For this review, take the finished solid that the model builds, in its own axes (mm). A direction names the side the tool comes from. Round coordinates to 2 decimals unless told otherwise and drop trailing zeros. Order: outer loops, then holes, each group sorted by start corner. A loop starts at its lowest first (then second) coordinate and runs counter-clockwise, first axis right, second up.
from build123d import *

# Parameters (mm, degrees)
BOSS_EXTRUDE1_DEPTH            = 8
CBORE_FOR_M5_SHCS1_D           = 5.5
CBORE_FOR_M5_SHCS1_DEPTH       = 8
CBORE_FOR_M5_SHCS1_CBORE_D     = 10.5
CBORE_FOR_M5_SHCS1_CBORE_DEPTH = 6


with BuildPart() as part:
    # Sketch1 → Boss-Extrude1 (new body)
    with BuildSketch(Plane(origin=(0, 0, 0), x_dir=(1, 0, 0), z_dir=(0, 1, 0))):
        with BuildLine():
            Line((3, 0), (37, 0))
            Line((37, 0), (40, 0))
            Line((40, 0), (40, 3))
            Line((40, 3), (40, 16))
            Line((40, 16), (25, 16))
            Line((25, 16), (25, 19))
            ThreePointArc((25, 19), (24.707106781, 19.707106781), (24, 20))
            Line((24, 20), (0, 20))
            Line((0, 20), (0, 3))
            ThreePointArc((0, 3), (0.878679656, 0.878679656), (3, 0))
        make_face()
    extrude(amount=BOSS_EXTRUDE1_DEPTH)

    # CBORE for M5 SHCS1
    with Locations(Plane(origin=(0, 8, 0), x_dir=(1, 0, 0), z_dir=(0, 1, 0))):
        with Locations((30, 10), (10, 10)):
            CounterBoreHole(CBORE_FOR_M5_SHCS1_D / 2, CBORE_FOR_M5_SHCS1_CBORE_D / 2, CBORE_FOR_M5_SHCS1_CBORE_DEPTH, depth=CBORE_FOR_M5_SHCS1_DEPTH)


solid = part.part
(1) Add section B-B on y = 7. Give the boundary of the cut face in (x, z).
(2) Add section A-A on x = 30. Give the boundary of the cut face in (y, z), plus the area to 3 significant figures.
(3) Add section D-D on y = 1.5. Give the boundary of the cut face in (x, z).
(4) Draft analysis for pull direction X (two halves, no side actions). For faces 4 (the face through (25, 4, -17)), 5 (the face through (20, 8, -10)), 6 (the face through (12.82, 5.04, -14.43)), state which applies: pulls with the +X half, pulls with the -X half, needs draft (parallel to the pull), parting line crosses it, or undercut.
(5) Add section C-C on x = 10. Give the boundary of the cut face in (y, z).
(6) Clearance check with flat-ended pins moving along their axes: P1, Ø8.5, axis at x = 30, z = -10, coming from the +Y side; P2, Ø4, axis at x = 34.5, y = 5.5, coming from the -Z side; P3, Ø1.5, axis at y = 3, z = -17, coming from the +X side. State where each tip first meets the part, or that it passes through.
(7) Tool access review of faces 1 (the face through (12, 4, -20)), 2 (the face through (26.13, 5.04, -13.55)), 3 (the face through (33, 4, -16)): name each direction out of +Z, -Z, +X, -X, +Y, -Y from which nothing blocks a thin tool from reaching the whole face with its end or side.
(8) Wall thickness on L1, parallel to X at y = 1.15, z = -10; L2, parallel to Z at x = 10, y = 1.5; L3, parallel to X at y = 2.5, z = -6.5: over which ranges is each line inside the solid? List them lowest first.
Here are the results:
1. outline: (0, -20) - (24, -20) arc R1 ccw to (25, -19) - (25, -16) - (40, -16) - (40, 0) - (3, 0) arc R3 ccw to (0, -3) - close; hole circle Ø10.5 at (10, -10); hole circle Ø10.5 at (30, -10)
2. outline: (0, -16) - (8, -16) - (8, -15.25) - (2, -15.25) - (2, -12.75) - (0, -12.75) - close; (0, -7.25) - (2, -7.25) - (2, -4.75) - (8, -4.75) - (8, 0) - (0, 0) - close
2. area: 54.0 mm2
3. outline: (0, -20) - (24, -20) arc R1 ccw to (25, -19) - (25, -16) - (40, -16) - (40, 0) - (3, 0) arc R3 ccw to (0, -3) - close; hole circle Ø5.5 at (10, -10); hole circle Ø5.5 at (30, -10)
4. face 4: pulls with the +X half
4. face 5: needs draft
4. face 6: undercut
5. outline: (0, -20) - (8, -20) - (8, -15.25) - (2, -15.25) - (2, -12.75) - (0, -12.75) - close; (0, -7.25) - (2, -7.25) - (2, -4.75) - (8, -4.75) - (8, 0) - (0, 0) - close
6. P1: stops at y = 2
6. P2: stops at z = -16
6. P3: stops at x = 25
7. face 1: -Z, +X, -X, +Y, -Y
7. face 2: +Y
7. face 3: -Z, +X, +Y, -Y
8. L1: x = 0 to 7.25, 12.75 to 27.25, 32.75 to 40
8. L2: z = -20 to -12.75, -7.25 to 0
8. L3: x = 0 to 6.09, 13.91 to 26.09, 33.91 to 40
